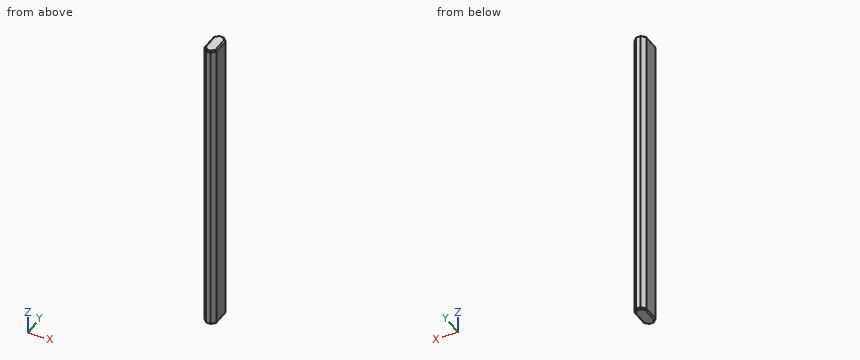
from build123d import *

# Parameters (mm, degrees)
ESBO_O2_W                = 4.7
ESBO_O2_H                = 9.7
RESSALTO_EXTRUS_O1_DEPTH = 119.7
CHANFRO1_SIZE            = 1.5
CHANFRO2_SIZE            = 0.5


with BuildPart() as part:
    # Esboço2 → Ressalto-extrusão1 (new body)
    with BuildSketch(Plane.XY):
        Rectangle(ESBO_O2_W, ESBO_O2_H)
    extrude(amount=RESSALTO_EXTRUS_O1_DEPTH)

    # Chanfro1
    chanfro1_edges = [part.edges().sort_by_distance(p)[0] for p in [
        (2.35, -4.85, 59.85),
        (-2.35, -4.85, 59.85),
        (-2.35, 4.85, 59.85),
        (2.35, 4.85, 59.85),
    ]]
    chamfer(chanfro1_edges, length=CHANFRO1_SIZE)

    # Chanfro2
    chanfro2_edges = [part.edges().sort_by_distance(p)[0] for p in [
        (0, -4.85, 0),
        (0, -4.85, 119.7),
        (2.35, 0, 0),
        (-2.35, 0, 0),
        (0, 4.85, 0),
        (1.6, 4.1, 0),
        (1.6, -4.1, 0),
        (-1.6, 4.1, 0),
        (-1.6, -4.1, 0),
        (-2.35, 0, 119.7),
        (2.35, 0, 119.7),
        (0, 4.85, 119.7),
        (1.6, 4.1, 119.7),
        (1.6, -4.1, 119.7),
        (-1.6, 4.1, 119.7),
        (-1.6, -4.1, 119.7),
    ]]
    chamfer(chanfro2_edges, length=CHANFRO2_SIZE)


solid = part.part
Read the model definition and answer for the solid it produces. Units are mm, in the model's axes. Round coordinates to 2 decimals unless told otherwise and drop trailing zeros. Loops run counter-clockwise (first coordinate to the right, second up) from the corner with the lowest first, then second, coordinate; pieces in that order, holes last.
Q1. This flat-tipped pin is pushed along its axis until it touches: pin 1 (1.5 mm diameter, centred on x = -2, z = 58, fed in from +Y). Where does it stop, or does it pass through?
Q2. Consider probe 1 along Z at (x, y) = (-1, -4); probe 2 along X at (y, z) = (-4.5, 14.5); probe 3 along X at (y, z) = (4, 21.5). Determine where each line is inside the solid, lowest interval first.
Q3. Section A-A on z = 68.5 is taken. Write down the section's boundary in (x, y).
Output:
1. pin 1: stops at y = 4.45
2. probe 1: z = 0.01 to 119.69
2. probe 2: x = -1.2 to 1.2
2. probe 3: x = -1.7 to 1.7
3. outline: (-2.35, -3.35) - (-0.85, -4.85) - (0.85, -4.85) - (2.35, -3.35) - (2.35, 3.35) - (0.85, 4.85) - (-0.85, 4.85) - (-2.35, 3.35) - close
